Check sheet for the modelled part. Datum: model origin and axes. Units: mm. Face numbers are marked on the shaded views. A direction names the side the tool comes from. Coordinates: 2 decimals unless noted, no trailing zeros. Order: outer loops, then holes, each group sorted by start corner. A loop starts at its lowest first (then second) coordinate and runs counter-clockwise, first axis right, second up.
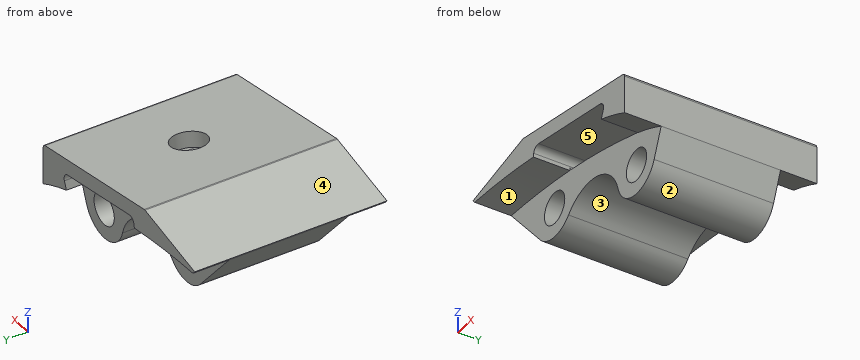
from build123d import *

# Parameters (mm, degrees)
F0_R     = 2.4
F1_DEPTH = 9
F2_DEPTH = 14.5
F3_R     = 0.5
F4_R     = 2.65
F5_DEPTH = 3


# Not quite as in the source:
# - two fillets or chamfers of one size are made in one step


with BuildPart() as f1:
    # F0 (on Front) → F1 (new body, symmetric)
    with BuildSketch(Plane.XZ):
        with BuildLine():
            Line((-19.2344364101, -14.475), (-12.351193111, -22.3932656305))
            ThreePointArc((-12.351193111, -22.3932656305), (-9.0297827018, -23.9403785735), (-5.6587929287, -22.5044978281))
            ThreePointArc((-5.6587929287, -22.5044978281), (1.0891796651, -20.5129837703), (6.0760796929, -25.4760564557))
            ThreePointArc((6.0760796929, -25.4760564557), (10.1567684842, -28.8420423371), (14.6192295456, -26.0015629336))
            Line((14.6192295456, -26.0015629336), (16.2763282151, -21.8))
            ThreePointArc((16.2763282151, -21.8), (13.5478934476, -20.5465737293), (10.7331243144, -19.5013424519))
            ThreePointArc((10.7331243144, -19.5013424519), (10.0239485931, -19.2751816233), (9.3106871937, -19.0622565188))
            ThreePointArc((9.3106871937, -19.0622565188), (2.0328204041, -17.1501268195), (-5.3587456661, -15.740043125))
            ThreePointArc((-5.3587456661, -15.740043125), (-12.2765411998, -14.887603878), (-19.2344364101, -14.475))
        make_face()
        with Locations((10.4330504183, -24.3505316455)):
            Circle(F0_R, mode=Mode.SUBTRACT)
        with Locations((-8.955, -19.441)):
            Circle(F0_R, mode=Mode.SUBTRACT)
        with BuildLine():
            Line((-19.6473476105, -14), (-19.2344364101, -14.475))
            ThreePointArc((-19.2344364101, -14.475), (-12.2765411998, -14.887603878), (-5.3587456661, -15.740043125))
            Line((-5.3587456661, -15.740043125), (-5.2650160599, -15.2084761138))
            ThreePointArc((-5.2650160599, -15.2084761138), (-4.8537847433, -14.5629722472), (-4.1065601293, -14.3973165385))
            Line((-4.1065601293, -14.3973165385), (10.4444975606, -16.9630606071))
            ThreePointArc((10.4444975606, -16.9630606071), (11.1434489978, -17.4594321695), (11.2011114112, -18.3147642019))
            Line((11.2011114112, -18.3147642019), (10.7331243144, -19.5013424519))
            ThreePointArc((10.7331243144, -19.5013424519), (13.5478934476, -20.5465737293), (16.2763282151, -21.8))
            Line((16.2763282151, -21.8), (16.2145160132, -15.6449893321))
            Line((16.2145160132, -15.6449893321), (-7.7940477934, -11.4116317649))
            Line((-7.7940477934, -11.4116317649), (-19.6473476105, -14))
        make_face()
    extrude(amount=F1_DEPTH, both=True)

    # F0 (on Front) → F2 (join, symmetric)
    with BuildSketch(Plane.XZ):
        with BuildLine():
            Line((-19.6473476105, -14), (-19.2344364101, -14.475))
            ThreePointArc((-19.2344364101, -14.475), (-12.2765411998, -14.887603878), (-5.3587456661, -15.740043125))
            Line((-5.3587456661, -15.740043125), (-5.2650160599, -15.2084761138))
            ThreePointArc((-5.2650160599, -15.2084761138), (-4.8537847433, -14.5629722472), (-4.1065601293, -14.3973165385))
            Line((-4.1065601293, -14.3973165385), (10.4444975606, -16.9630606071))
            ThreePointArc((10.4444975606, -16.9630606071), (11.1434489978, -17.4594321695), (11.2011114112, -18.3147642019))
            Line((11.2011114112, -18.3147642019), (10.7331243144, -19.5013424519))
            ThreePointArc((10.7331243144, -19.5013424519), (13.5478934476, -20.5465737293), (16.2763282151, -21.8))
            Line((16.2763282151, -21.8), (16.2145160132, -15.6449893321))
            Line((16.2145160132, -15.6449893321), (-7.7940477934, -11.4116317649))
            Line((-7.7940477934, -11.4116317649), (-19.6473476105, -14))
        make_face()
    extrude(amount=F2_DEPTH, both=True)

    # F3
    f3_edges = [f1.edges().sort_by_distance(p)[0] for p in [
        (-5.358746, 0, -15.740043),
        (10.733124, 0, -19.501342),
        (16.214516, 0, -15.644989),
        (-7.794048, 0, -11.411632),
    ]]
    fillet(f3_edges, radius=F3_R)

    # F4 (on face) → F5 (cut)
    with BuildSketch(Plane(origin=(-2.1865232639, 0, -12.4003896345), x_dir=(0.984807753, 0, -0.1736481777), z_dir=(0.1736481777, 0, 0.984807753))):
        with Locations((6.7739703659, 0)):
            Circle(F4_R)
    extrude(amount=-F5_DEPTH, mode=Mode.SUBTRACT)


solid = f1.part
(1) Release check for a two-part mould opening along Z. For the marked faces 3, 4 and 5 record: +Z half, -Z half, draft (parallel to the pull), parting line (faces both ways), or undercut.
Filled in:
face 3: -Z half
face 4: +Z half
face 5: undercut
(2) Thickness scan on probe 1 along Z at (x, y) = (-8, -5.75); probe 2 along X at (y, z) = (-0.5, -15.75); probe 3 along Y at (x, z) = (13.5, -21.75). Record the ranges inside material, lowest first.
Filled in:
probe 1: z = -23.84 to -21.64, -17.24 to -11.46
probe 2: x = -18.13 to -5.04, 6.74 to 16.11
probe 3: y = -9 to 9
(3) Cross-section at C-C (x = -15). Enter the section's corners in (y, z), and give its area (3 significant figures).
Filled in:
outline: (-14.5, -14.67) - (-9, -14.67) - (-9, -19.35) - (9, -19.35) - (9, -14.67) - (14.5, -14.67) - (14.5, -12.99) - (-14.5, -12.99) - close
area: 133 mm2
(4) Cross-section at B-B (y = 1.5). Count the separate pieces of the cut face and the enclosed holes in it, and give its area (3 significant figures).
Filled in:
separate pieces: 1
enclosed holes: 2
area: 267 mm2
(5) Go/stop test with flat-tipped pins: P1, Ø5, axis at x = -15.5, z = -18, coming from the -Y side; P2, Ø3, axis at x = 1, y = 7, coming from the -Z side; P3, Ø3, axis at x = -1, y = -4.5, coming from the +Z side; P4, Ø3, axis at x = -8.955, z = -19.441, coming from the +Y side. Record where each tip stops, or that it passes through.
Filled in:
P1: stops at y = -9
P2: stops at z = -21.04
P3: stops at z = -12.35
P4: passes through
(6) Tool access check on the marked faces 1 and 2. Record the directions out of +Z, -Z, +X, -X, +Y, -Y that give a thin tool (end or side, any length) a straight path to the whole face; none if there is none.
Filled in:
face 1: -Z, -X, -Y
face 2: -Z, +Y, -Y
